```python
from build123d import *

# Parameters (mm, degrees)
SKETCH1_W           = 76.2
SKETCH1_H           = 12.7
BOSS_EXTRUDE1_DEPTH = 3.175
SKETCH4_W           = 3.175
SKETCH4_H           = 6.35
CUT_EXTRUDE1_DEPTH  = 4.175
LPATTERN1_COUNT     = 4
LPATTERN1_PITCH     = 15.875


with BuildPart() as part:
    # Sketch1 → Boss-Extrude1 (new body)
    with BuildSketch(Plane(origin=(0, 0, 0), x_dir=(1, 0, 0), z_dir=(0, 1, 0))):
        with Locations((38.1, -6.35)):
            Rectangle(SKETCH1_W, SKETCH1_H)
    extrude(amount=BOSS_EXTRUDE1_DEPTH)

    # Sketch4 → Cut-Extrude1 (cut, through all)
    with BuildSketch(Plane(origin=(0, 3.175, 0), x_dir=(1, 0, 0), z_dir=(0, 1, 0))):
        with Locations((14.2875, -9.525)):
            Rectangle(SKETCH4_W, SKETCH4_H)
    cut_extrude1 = extrude(amount=-CUT_EXTRUDE1_DEPTH, mode=Mode.SUBTRACT)

    # LPattern1: Cut-Extrude1 ×4
    with Locations(*[(i * LPATTERN1_PITCH, 0, 0) for i in range(1, LPATTERN1_COUNT)]):
        add(cut_extrude1, mode=Mode.SUBTRACT)


solid = part.part
```
For this review, take the finished solid that the model builds, in its own axes (mm). A direction names the side the tool comes from. Coordinates: 2 decimals unless noted, no trailing zeros. Write each loop counter-clockwise with the first axis right and the second up, starting at its lowest first coordinate (ties: lowest second). Pieces come first, ordered by that corner, then holes.
(1) Tool access review of faces 4 (the face through (38, 3.175, 6)), 5 (the face through (31.75, 2, 10)): name each direction out of +Z, -Z, +X, -X, +Y, -Y from which nothing blocks a thin tool from reaching the whole face with its end or side.
(2) Add section C-C on x = 61.5. Give the boundary of the cut face in (y, z) (3 decimals).
(3) Add section B-B on y = 1.2. Give the boundary of the cut face in (x, z) (3 decimals), then the cut area to 3 significant figures.
(4) The part is to be moulded in two halves that separate along X. For faces 1 (the face through (54, 2, 12.7)), 2 (the face through (76.2, 2, 6)), 3 (the face through (62, 2, 6.35)), say which applies: +X half, -X half, draft (parallel to the pull), parting line (faces both ways), or undercut.
(5) Add section A-A on z = 8.75. Give the boundary of the cut face in (x, y) (3 decimals), then the cut area to 3 significant figures.
(6) Wall thickness on probe 1 along X at (y, z) = (0.75, 11) (3 decimals); probe 2 along Z at (x, y) = (60.5, 1.1): over which ranges is each line inside the solid? List them lowest first.
Answer sheet:
1. face 4: +Z, -Z, +X, -X, +Y
1. face 5: +Z, +Y, -Y
2. outline: (0, 0) - (3.175, 0) - (3.175, 6.35) - (0, 6.35) - close
3. outline: (0, 0) - (76.2, 0) - (76.2, 12.7) - (63.5, 12.7) - (63.5, 6.35) - (60.325, 6.35) - (60.325, 12.7) - (47.625, 12.7) - (47.625, 6.35) - (44.45, 6.35) - (44.45, 12.7) - (31.75, 12.7) - (31.75, 6.35) - (28.575, 6.35) - (28.575, 12.7) - (15.875, 12.7) - (15.875, 6.35) - (12.7, 6.35) - (12.7, 12.7) - (0, 12.7) - close
3. area: 887 mm2
4. face 1: draft
4. face 2: +X half
4. face 3: undercut
5. outline: (0, 0) - (12.7, 0) - (12.7, 3.175) - (0, 3.175) - close; (15.875, 0) - (28.575, 0) - (28.575, 3.175) - (15.875, 3.175) - close; (31.75, 0) - (44.45, 0) - (44.45, 3.175) - (31.75, 3.175) - close; (47.625, 0) - (60.325, 0) - (60.325, 3.175) - (47.625, 3.175) - close; (63.5, 0) - (76.2, 0) - (76.2, 3.175) - (63.5, 3.175) - close
5. area: 202 mm2
6. probe 1: x = 0 to 12.7, 15.875 to 28.575, 31.75 to 44.45, 47.625 to 60.325, 63.5 to 76.2
6. probe 2: z = 0 to 6.35
